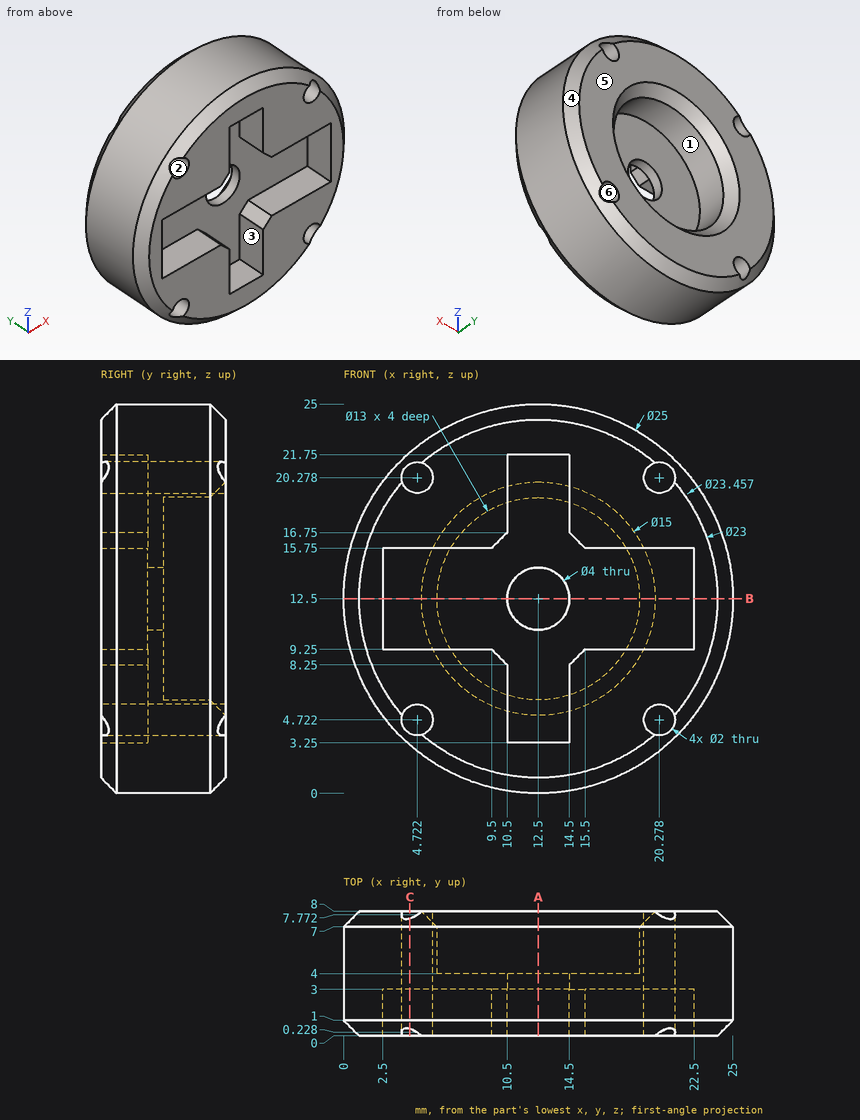
The figure shows three views and two pictorial views of one solid part (mm, origin at its lowest corner). Answer the questions. A direction names the side the tool comes from. Give positions to 0.01 mm unless a question says otherwise; leave off trailing zeros. Order: outer loops, then holes, each group sorted by start corner. A loop starts at its lowest first (then second) coordinate and runs counter-clockwise, first axis right, second up. Notation, with made-up numbers: (-2, 77) -> (30, 77) arc R10 ccw to (30, 83) -> close; hole circle Ø2 at (79, -26). An arc over 180 degrees is marked (long way). Answer as a JSON object with one key per item and string values. Group by question number.
Item 1: The part is cut by section B-B on z = 12.5. Write down the section's boundary in (x, y).
Item 2: Determine the mould class of the marked faces 4, 5 and 6 for opening direction X: pulls with the +X half, pulls with the -X half, needs draft (parallel to the pull), parting line crosses it, or undercut.
Item 3: The part is cut by section A-A on x = 12.5. Write down the section's boundary in (y, z).
Item 4: Consider L1, parallel to Z at x = 4.75, y = 1.5; L2, parallel to Z at x = 4.75, y = 4.25; L3, parallel to X at y = 2.75, z = 15.25 (1 decimal). Determine where each line is inside the solid, lowest interval first. Write a range as from..to.
Item 5: A tool of negligible diameter and unlimited length cuts with its end or side. For the marked faces 1, 2 and 3, from which of +Z, -Z, +X, -X, +Y, -Y can it reach the whole face along a straight path? Write none if from no direction.
Item 6: Flat-ended cylindrical pins translate along their axes: pin 1 (2.5 mm diameter, centred on x = 19, y = 2, fed in from -Z) (1 decimal); pin 2 (2.5 mm diameter, centred on y = 1.5, z = 19, fed in from +X) (1 decimal); pin 3 (3.5 mm diameter, centred on y = 2, z = 4.5, fed in from +X) (1 decimal); pin 4 (1.6 mm diameter, centred on x = 4.72, z = 4.72, fed in from -Y). Find the tip coordinate at first contact, or state that the pin passes through.
Item 7: The part is cut by section C-C on x = 4.25. Give the number of separate pieces and of enclosed holes in the cut face, and give its area (3 significant figures).
Result set:
{
 "1": {"outline": "(0, 1) -> (1, 0) -> (2.5, 0) -> (2.5, 3) -> (10.5, 3) -> (10.5, 4) -> (6, 4) -> (6, 7) -> (5, 8) -> (1, 8) -> (0, 7) -> close; (14.5, 3) -> (22.5, 3) -> (22.5, 0) -> (24, 0) -> (25, 1) -> (25, 7) -> (24, 8) -> (20, 8) -> (19, 7) -> (19, 4) -> (14.5, 4) -> close"},
 "2": {"face 4": "parting line crosses it", "face 5": "needs draft", "face 6": "undercut"},
 "3": {"outline": "(0, 1) -> (1, 0) -> (7, 0) -> (8, 1) -> (8, 5) -> (7, 6) -> (4, 6) -> (4, 10.5) -> (3, 10.5) -> (3, 3.25) -> (0, 3.25) -> close; (0, 21.75) -> (3, 21.75) -> (3, 14.5) -> (4, 14.5) -> (4, 19) -> (7, 19) -> (8, 20) -> (8, 24) -> (7, 25) -> (1, 25) -> (0, 24) -> close"},
 "4": {"L1": "2.69..3.72, 5.72..9.25, 15.75..19.28, 21.28..22.31", "L2": "2.69..3.72, 5.72..19.28, 21.28..22.31", "L3": "0.3..2.5, 22.5..24.7"},
 "5": {"face 1": "+Y", "face 2": "+Y, -Y", "face 3": "-Y"},
 "6": {"pin 1": "z = 1.2", "pin 2": "x = 23.8", "pin 3": "x = 23.3", "pin 4": "through"},
 "7": {"separate pieces": "3", "enclosed holes": "0", "area": "100 mm²"}
}
